Read the model definition and answer for the solid it produces. Units are mm, in the model's axes. Face numbers are marked on the shaded views. A direction names the side the tool comes from. Round coordinates to 2 decimals unless told otherwise and drop trailing zeros. Loops run counter-clockwise (first coordinate to the right, second up) from the corner with the lowest first, then second, coordinate; pieces in that order, holes last. Notation, with made-up numbers: (33.25, 40) -> (56.25, 40) arc R12 ccw to (56.25, 47) -> close; hole circle Ø11 at (-2.5, 62.5). An arc over 180 degrees is marked (long way). Put each result on its own line as item: value.
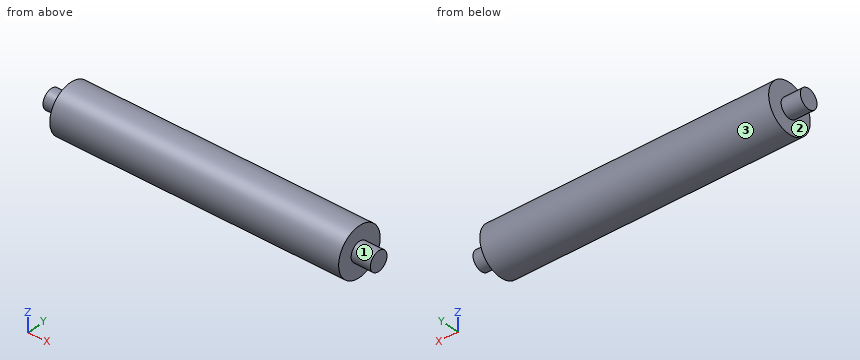
Autodesk Inventor part; units mm, degrees
ref_plane "YZ Plane" through (0, 0, 0) normal (1, 0, 0) x (0, 1, 0)
ref_plane "XZ Plane" through (0, 0, 0) normal (0, 1, 0) x (-1, 0, 0)
ref_plane "XY Plane" through (0, 0, 0) normal (0, 0, 1) x (1, 0, 0)
sketch "Sketch1" plane through (0, 0, 0) normal (1, 0, 0) x (0, 1, 0)
  circle A0 centre (0, 0) radius 12.5
  dimension "d0" = 25
extrude "Extrusion1" add sketch "Sketch1" along normal blind 170
sketch "Sketch2" plane through (170, 0, 0) normal (1, 0, 0) x (0, 0, -1)
  circle A0 centre (0, 0) radius 12.5
  dimension "d3" = 25
extrude "Extrusion2" cut sketch "Sketch2" against normal blind 10
sketch "Sketch3" plane through (160, 0, 0) normal (1, 0, 0) x (0, 0, -1)
  circle A0 centre (0, 0) radius 5
  dimension "d6" = 10
extrude "Extrusion3" add sketch "Sketch3" along normal blind 10
sketch "Sketch4" plane through (0, 0, 0) normal (-1, 0, 0) x (0, 0, 1)
  circle A0 centre (0, 0) radius 12.5
  dimension "d9" = 25
extrude "Extrusion4" cut sketch "Sketch4" against normal blind 10
sketch "Sketch5" plane through (10, 0, 0) normal (-1, 0, 0) x (0, 0, 1)
  circle A0 centre (0, 0) radius 5
  circle A1 centre (0, 0) radius 5
extrude "Extrusion5" add sketch "Sketch5" along normal blind 10
properties part number "laser" material "Glass"
Item 1: The part is cut by section D-D (z = -10). Determine the outline of the cut face in (x, y), then the cut area to 3 significant figures.
Derived:
outline: (10, -7.5) -> (160, -7.5) -> (160, 7.5) -> (10, 7.5) -> close
area: 2,250 mm^2
Item 2: The part is cut by section C-C (x = 41). Determine the outline of the cut face in (y, z).
Derived:
outline: circle Ø25 at (0, 0)
Item 3: Which of the six approach directions +Z, -Z, +X, -X, +Y, -Y give full straight-line access (tool end or side, diameter ignored) to the marked faces 1, 2 and 3?
Derived:
face 1: +X
face 2: -X
face 3: +X, -X
Item 4: Flat-ended cylindrical pins translate along their axes: pin 1 Ø8 at (x, z) = (101, -6) entering from -Y; pin 2 Ø1 at (x, y) = (111.5, 5.5) entering from -Z; pin 3 Ø6 at (x, y) = (106.5, -4.5) entering from -Z. Find the tip coordinate at first contact, or state that the pin passes through.
Derived:
pin 1: stops at y = -12.34
pin 2: stops at z = -11.46
pin 3: stops at z = -12.41
Item 5: The part is cut by section A-A (y = 0). Determine the outline of the cut face in (x, z).
Derived:
outline: (0, -5) -> (10, -5) -> (10, -12.5) -> (160, -12.5) -> (160, -5) -> (170, -5) -> (170, 5) -> (160, 5) -> (160, 12.5) -> (10, 12.5) -> (10, 5) -> (0, 5) -> close
Item 6: Find the intervals of material crossed by line 1 along X through (y, z) = (6, -7.25); line 2 along Z through (x, y) = (99, -0.5), in increasing order.
Derived:
line 1: x = 10 to 160
line 2: z = -12.49 to 12.49
